```python
from build123d import *

# Parameters (mm, degrees)
F0_W      = 42.3
F0_H      = 42.3
F1_DEPTH  = 39
F2_R      = 11
F3_DEPTH  = 2
F4_R      = 1.5
F5_DEPTH  = 4.5
F6_R      = 1.5
F7_DEPTH  = 4.5
F8_R      = 1.5
F9_DEPTH  = 4.5
F10_R     = 1.5
F11_DEPTH = 4.5
F12_R     = 5
F13_DEPTH = 5
F14_R     = 2.5
F15_DEPTH = 27


with BuildPart() as f1:
    # F0 (on Top) → F1 (new body)
    with BuildSketch(Plane.XY):
        Rectangle(F0_W, F0_H)
    extrude(amount=F1_DEPTH)

    # F2 (on face) → F3 (join)
    with BuildSketch(Plane.XY.offset(39)):
        Circle(F2_R)
    extrude(amount=F3_DEPTH)

    # F4 (on face) → F5 (cut)
    with BuildSketch(Plane.XY.offset(39)):
        with Locations((15.65, 15.65)):
            Circle(F4_R)
    extrude(amount=-F5_DEPTH, mode=Mode.SUBTRACT)

    # F6 (on face) → F7 (cut)
    with BuildSketch(Plane.XY.offset(39)):
        with Locations((15.65, -15.65)):
            Circle(F6_R)
    extrude(amount=-F7_DEPTH, mode=Mode.SUBTRACT)

    # F8 (on face) → F9 (cut)
    with BuildSketch(Plane.XY.offset(39)):
        with Locations((-15.65, -15.65)):
            Circle(F8_R)
    extrude(amount=-F9_DEPTH, mode=Mode.SUBTRACT)

    # F10 (on face) → F11 (cut)
    with BuildSketch(Plane.XY.offset(39)):
        with Locations((-15.65, 15.65)):
            Circle(F10_R)
    extrude(amount=-F11_DEPTH, mode=Mode.SUBTRACT)

    # F12 (on face) → F13 (cut)
    with BuildSketch(Plane.XY.offset(41)):
        Circle(F12_R)
    extrude(amount=-F13_DEPTH, mode=Mode.SUBTRACT)

    # F14 (on face) → F15 (join)
    with BuildSketch(Plane.XY.offset(36)):
        Circle(F14_R)
    extrude(amount=F15_DEPTH)


solid = f1.part
```
The listing builds one solid part. Answer for the finished solid, in the listing's coordinates (mm). A direction names the side the tool comes from. Coordinates: 2 decimals unless noted, no trailing zeros. Write each loop counter-clockwise with the first axis right and the second up, starting at its lowest first coordinate (ties: lowest second). Pieces come first, ordered by that corner, then holes. Notation, with made-up numbers: (-37.5, 52.25) - (21.5, 52.25) arc R31 cw to (21.5, 85.25) - close; hole circle Ø9 at (-25, 86.25). An arc over 180 degrees is marked (long way). Return JSON: item names as keys, results as strings. Group by question number.
1. Which of the six approach directions +Z, -Z, +X, -X, +Y, -Y give full straight-line access (tool end or side, diameter ignored) to faces 4 (the flat face through (-16, -16, 34.5)), 5 (the flat face through (0, 0, 63))?
2. A cutting plane is placed at D-D, the plane x = -15.65. Determine the outline of the cut face in (y, z).
3. A cutting plane is placed at B-B, the plane x = 0. Determine the outline of the cut face in (y, z), plus the area to 3 significant figures.
4. Determine the mould class of faces 1 (the cylindrical face through (15.455, -14.163, 36.782)), 2 (the flat face through (-21.15, 0, 19)), 3 (the flat face through (0, -21.15, 19)) for opening direction X: released by +X, released by -X, zero draft, split by the parting line, or undercut.
5. Straight lines are drawn through the part: L1, parallel to Y at x = -15.65, z = 36.7; L2, parallel to Y at x = 0, z = 38; L3, parallel to X at y = -15, z = 37. For each, find the intervals that lie inside material, in ascending order.
6. A cutting plane is placed at A-A, the plane z = 37. Determine the outline of the cut face in (x, y).
7. Given pin 1 (0.9 mm diameter, centred on x = -16, y = -15.5, fed in from +Z); pin 2 (3.5 mm diameter, centred on x = 15.65, y = 15.65, fed in from +Z); pin 3 (10 mm diameter, centred on x = -15, z = 47, fed in from +Y); pin 4 (1.5 mm diameter, centred on y = 2, z = 47, fed in from -X), each flat-ended and moving along its own axis, determine where each tip first touches the part or whether it passes through.
Ans:
{
 "1": {"face 4": "+Z", "face 5": "+Z, +X, -X, +Y, -Y"},
 "2": {"outline": "(-21.15, 0) - (21.15, 0) - (21.15, 39) - (17.15, 39) - (17.15, 34.5) - (14.15, 34.5) - (14.15, 39) - (-14.15, 39) - (-14.15, 34.5) - (-17.15, 34.5) - (-17.15, 39) - (-21.15, 39) - close"},
 "3": {"outline": "(-21.15, 0) - (21.15, 0) - (21.15, 39) - (11, 39) - (11, 41) - (5, 41) - (5, 36) - (2.5, 36) - (2.5, 63) - (-2.5, 63) - (-2.5, 36) - (-5, 36) - (-5, 41) - (-11, 41) - (-11, 39) - (-21.15, 39) - close", "area": "1,780 mm²"},
 "4": {"face 1": "undercut", "face 2": "released by -X", "face 3": "zero draft"},
 "5": {"L1": "-21.15 to -17.15, -14.15 to 14.15, 17.15 to 21.15", "L2": "-21.15 to -5, -2.5 to 2.5, 5 to 21.15", "L3": "-21.15 to -17, -14.3 to 14.3, 17 to 21.15"},
 "6": {"outline": "(-21.15, -21.15) - (21.15, -21.15) - (21.15, 21.15) - (-21.15, 21.15) - close; circle Ø5 at (0, 0); hole circle Ø3 at (-15.65, -15.65); hole circle Ø3 at (-15.65, 15.65); hole circle Ø10 at (0, 0); hole circle Ø3 at (15.65, -15.65); hole circle Ø3 at (15.65, 15.65)"},
 "7": {"pin 1": "z = 34.5", "pin 2": "z = 39", "pin 3": "through", "pin 4": "x = -2.17"}
}
